Work out the finished part from the listing and answer in its coordinate system (mm). A direction names the side the tool comes from. Coordinates: 2 decimals unless noted, no trailing zeros. Loops run counter-clockwise (first coordinate to the right, second up) from the corner with the lowest first, then second, coordinate; pieces in that order, holes last. Notation, with made-up numbers: (79.25, 10.25) -> (121.25, 10.25) arc R31 cw to (121.25, 42.25) -> close; hole circle Ø1 at (8, -5.5). An arc over 180 degrees is marked (long way). Use a Markdown table: item, result. Add a question column.
```python
from build123d import *

# Parameters (mm, degrees)
SKETCH1_R               = 15
BOSS_EXTRUDE1_DEPTH     = 3
BOSS_EXTRUDE2_START     = -1.5
SKETCH2_R               = 1.6
BOSS_EXTRUDE2_DEPTH     = 1.5
MIRROR2_START           = -1.5
MIRROR2_COPY_1_SKETCH_R = 1.6
MIRROR2_COPY_1_DEPTH    = 1.5
SKETCH3_R               = 5
BOSS_EXTRUDE3_DEPTH     = 8
CHAMFER1_SIZE           = 5
SKETCH5_R               = 1.7
CUT_EXTRUDE1_DEPTH      = 12


with BuildPart() as part:
    # Sketch1 → Boss-Extrude1 (new body)
    with BuildSketch(Plane.XY):
        Circle(SKETCH1_R)
    extrude(amount=BOSS_EXTRUDE1_DEPTH)

    # Sketch2 → Boss-Extrude2 (add, symmetric)
    with BuildSketch(Plane.XY.offset(3).offset(BOSS_EXTRUDE2_START)):
        with BuildLine():
            Line((-18.163571809, 12.764485711), (-14.497712513, 3.849198865))
            ThreePointArc((-14.497712513, 3.849198865), (-10.606601718, 10.606601718), (-3.849198865, 14.497712513))
            Line((-3.849198865, 14.497712513), (-12.764485711, 18.163571809))
            ThreePointArc((-12.764485711, 18.163571809), (-17.262762767, 17.262762767), (-18.163571809, 12.764485711))
        make_face()
        with Locations((-14.33765637, 14.33765637)):
            Circle(SKETCH2_R, mode=Mode.SUBTRACT)
    boss_extrude2 = extrude(amount=BOSS_EXTRUDE2_DEPTH, both=True)

    # Mirror1: Boss-Extrude2 across plane
    add(boss_extrude2.mirror(Plane(origin=(0, 0, 0), x_dir=(0, 0, 1), z_dir=(1, 0, 0))))

    # Mirror2: Boss-Extrude2 across plane
    add(boss_extrude2.mirror(Plane.ZX))

    # Mirror2 copy 1 sketch → Mirror2 copy 1 (add, symmetric)
    with BuildSketch(Plane(origin=(0, 0, 3), x_dir=(-1, 0, 0), z_dir=(0, 0, 1)).offset(MIRROR2_START)):
        with BuildLine():
            Line((-18.163571809, 12.764485711), (-14.497712513, 3.849198865))
            ThreePointArc((-14.497712513, 3.849198865), (-10.606601718, 10.606601718), (-3.849198865, 14.497712513))
            Line((-3.849198865, 14.497712513), (-12.764485711, 18.163571809))
            ThreePointArc((-12.764485711, 18.163571809), (-17.262762767, 17.262762767), (-18.163571809, 12.764485711))
        make_face()
        with Locations((-14.33765637, 14.33765637)):
            Circle(MIRROR2_COPY_1_SKETCH_R, mode=Mode.SUBTRACT)
    extrude(amount=MIRROR2_COPY_1_DEPTH, both=True)

    # Sketch3 → Boss-Extrude3 (add)
    with BuildSketch(Plane.XY.offset(3)):
        Circle(SKETCH3_R)
    extrude(amount=BOSS_EXTRUDE3_DEPTH)

    # Sketch4 → Revolve1 (revolve)
    with BuildSketch(Plane(origin=(0, 0, 0), x_dir=(1, 0, 0), z_dir=(0, 1, 0))):
        Polygon((0, -11), (-5, -11), (-2.5, -17), (0, -17), align=None)
    revolve(axis=Axis((0, 0, 11), (0, 0, 1)))

    # Chamfer1
    chamfer1_edges = [part.edges().sort_by_distance(p)[0] for p in [
        (-5, 0, 3),
    ]]
    chamfer(chamfer1_edges, length=CHAMFER1_SIZE)

    # Sketch5 → Cut-Extrude1 (cut)
    with BuildSketch(Plane.XY.offset(17)):
        Circle(SKETCH5_R)
    extrude(amount=-CUT_EXTRUDE1_DEPTH, mode=Mode.SUBTRACT)


solid = part.part
```
Item 1: Find the intervals of material crossed by probe 1 along Z at (x, y) = (0.5, -14); probe 2 along Y at (x, z) = (3, 10); probe 3 along Z at (x, y) = (-5, 2.5), in increasing order.
Item 2: Section B-B (y = 0) is taken. Determine the outline of the cut face in (x, z), then the cut area to 3 significant figures.
Item 3: Section A-A (x = 14) is taken. Determine the outline of the cut face in (y, z).
Item 4: For a pull along Y with two mould halves and no side action, classify faces 4 (the face through (16.356, 8.369, 1.521)), 5 (the face through (8.244, -16.305, 1.521)), 6 (the face through (-2, 1, 17)) as +Y half, -Y half, draft (parallel to the pull), parting line (faces both ways), or undercut.
Item 5: For faces 1 (the face through (-16.356, -8.369, 1.521)), 2 (the face through (-8.244, 16.305, 1.521)), 3 (the face through (13.5, -15.7, 1.5)), determine the directions among +Z, -Z, +X, -X, +Y, -Y from which every point of the face is accessible in a straight line to the end or side of a thin tool.
Item 6: Given pin 1 (3 mm diameter, centred on x = 5.5, z = 10, fed in from -Y); pin 2 (1 mm diameter, centred on x = 12.5, y = -10.5, fed in from +Z); pin 3 (6 mm diameter, centred on x = 4.5, z = 14, fed in from -Y); pin 4 (1.9 mm diameter, centred on x = 14.34, y = -14.34, fed in from -Z), each flat-ended and moving along its own axis, determine where each tip first touches the part or whether it passes through.
Item 7: Section C-C (z = 6.5) is taken. Determine the outline of the cut face in (x, y).
Output:
| question | item | result |
|---|---|---|
| 1 | probe 1 | z = 0 to 3 |
| 1 | probe 2 | y = -4 to 4 |
| 1 | probe 3 | z = 0 to 7.41 |
| 2 | outline | (-15, 0) -> (15, 0) -> (15, 3) -> (10, 3) -> (5, 8) -> (5, 11) -> (2.5, 17) -> (1.7, 17) -> (1.7, 5) -> (-1.7, 5) -> (-1.7, 17) -> (-2.5, 17) -> (-5, 11) -> (-5, 8) -> (-10, 3) -> (-15, 3) -> close |
| 2 | area | 199 mm2 |
| 3 | outline | (-18.46, 0) -> (-15.9, 0) -> (-15.9, 3) -> (-18.46, 3) -> close; (-12.77, 0) -> (12.77, 0) -> (12.77, 3) -> (-12.77, 3) -> close; (15.9, 0) -> (18.46, 0) -> (18.46, 3) -> (15.9, 3) -> close |
| 4 | face 4 | undercut |
| 4 | face 5 | -Y half |
| 4 | face 6 | draft |
| 5 | face 1 | +Z, -Z, -X |
| 5 | face 2 | +Z, -Z, +Y |
| 5 | face 3 | +Z, -Z |
| 6 | pin 1 | stops at y = -3 |
| 6 | pin 2 | stops at z = 3 |
| 6 | pin 3 | stops at y = -3.99 |
| 6 | pin 4 | passes through |
| 7 | outline | circle Ø13 at (0, 0); hole circle Ø3.4 at (0, 0) |
